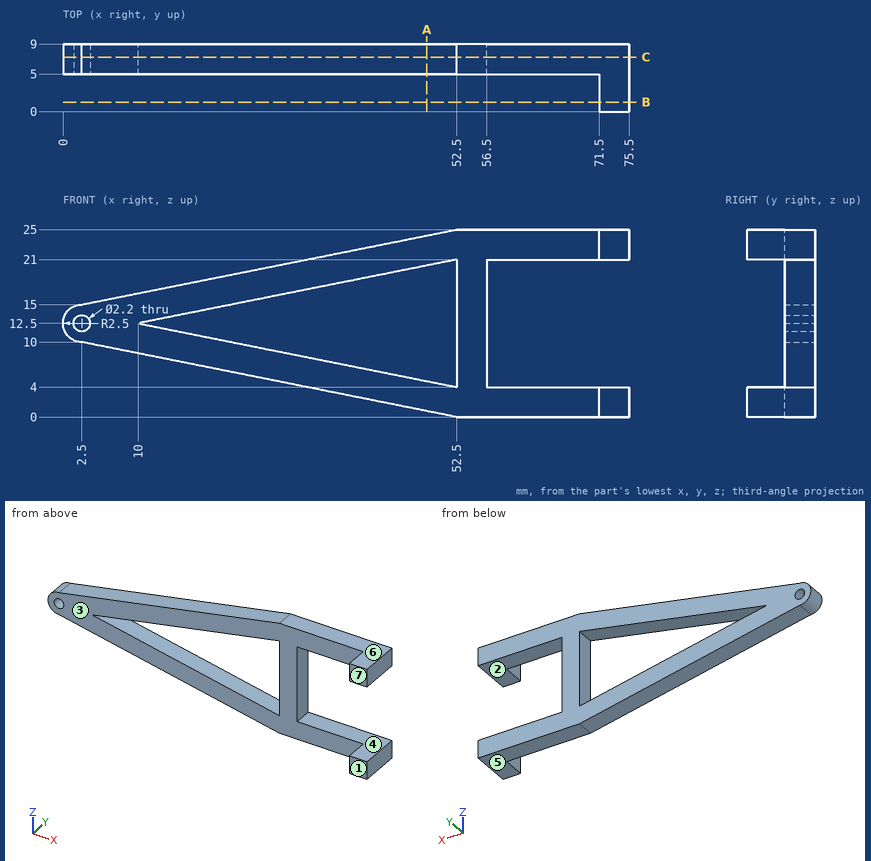
Verification items for this drawing (mm, ordinates from the low corner). A direction names the side the tool comes from. Give positions to 0.01 mm unless a question says otherwise; leave off trailing zeros. Loops run counter-clockwise (first coordinate to the right, second up) from the corner with the lowest first, then second, coordinate; pieces in that order, holes last. Notation, with made-up numbers: M 86,-31.75 L 116,-31.75 A16 ccw 116,-6.75 Z; hole C 68.25,-23 d9. An arc over 180 degrees is marked long. Answer in a Markdown table with one row per item.
1) Cross-section at A-A (x = 48.5). Enter the section's corners in (y, z), plus the area to 3 significant figures.
Solutions:
| item | result |
|---|---|
| outline | M 5,0.8 L 9,0.8 L 9,4.8 L 5,4.8 Z; M 5,20.2 L 9,20.2 L 9,24.2 L 5,24.2 Z |
| area | 32.0 mm^2 |
2) Cross-section at C-C (y = 7.25). Enter the section's corners in (x, z), plus the area to 3 significant figures.
Solutions:
| item | result |
|---|---|
| outline | M 2.5,10 L 52.5,0 L 75.5,0 L 75.5,4 L 56.5,4 L 56.5,21 L 75.5,21 L 75.5,25 L 52.5,25 L 2.5,15 A2.5 ccw Z; hole C 2.5,12.5 d2.2; hole M 10,12.5 L 52.5,4 L 52.5,21 Z |
| area | 647 mm^2 |
3) Depth check by flat-ended pin: pin 1 (4 mm diameter, centred on x = 26.5, z = 4, fed in from +Y); pin 2 (2 mm diameter, centred on y = 2, z = 1.5, fed in from -X); pin 3 (2 mm diameter, centred on y = 8, z = 14.5, fed in from -X); pin 4 (12.5 mm diameter, centred on x = 49.5, z = 18.5, fed in from -Y). Enter the tip coordinate at first touch or a pass-through.
Solutions:
| item | result |
|---|---|
| pin 1 | stops at y = 9 |
| pin 2 | stops at x = 71.5 |
| pin 3 | stops at x = 0.21 |
| pin 4 | stops at y = 5 |
4) Cross-section at B-B (y = 1.25). Enter the section's corners in (x, z), plus the area to 3 significant figures.
Solutions:
| item | result |
|---|---|
| outline | M 71.5,0 L 75.5,0 L 75.5,4 L 71.5,4 Z; M 71.5,21 L 75.5,21 L 75.5,25 L 71.5,25 Z |
| area | 32.0 mm^2 |
5) Thickness scan on line 1 (Z direction, x = 2.5, y = 6.3); line 2 (Z direction, x = 47.5, y = 7.75); line 3 (Y direction, x = 54, z = 4). Record the ranges inside material, lowest first.
Solutions:
| item | result |
|---|---|
| line 1 | z = 10 to 11.4, 13.6 to 15 |
| line 2 | z = 1 to 5, 20 to 24 |
| line 3 | y = 5 to 9 |
6) Tool access check on the marked faces 1, 2 and 3. Record the directions out of +Z, -Z, +X, -X, +Y, -Y that give a thin tool (end or side, any length) a straight path to the whole face; none if there is none.
Solutions:
| item | result |
|---|---|
| face 1 | +Z, -Z, +X, -X, -Y |
| face 2 | +X, +Y, -Y |
| face 3 | +Z, -Z, -X, -Y |
7) Mould release check, pull along Z, two halves, no side actions. Record for the marked faces 4, 5, 6 and 7: released by +Z, released by -Z, zero draft, split by the parting line, or undercut.
Solutions:
| item | result |
|---|---|
| face 4 | undercut |
| face 5 | released by -Z |
| face 6 | released by +Z |
| face 7 | zero draft |
